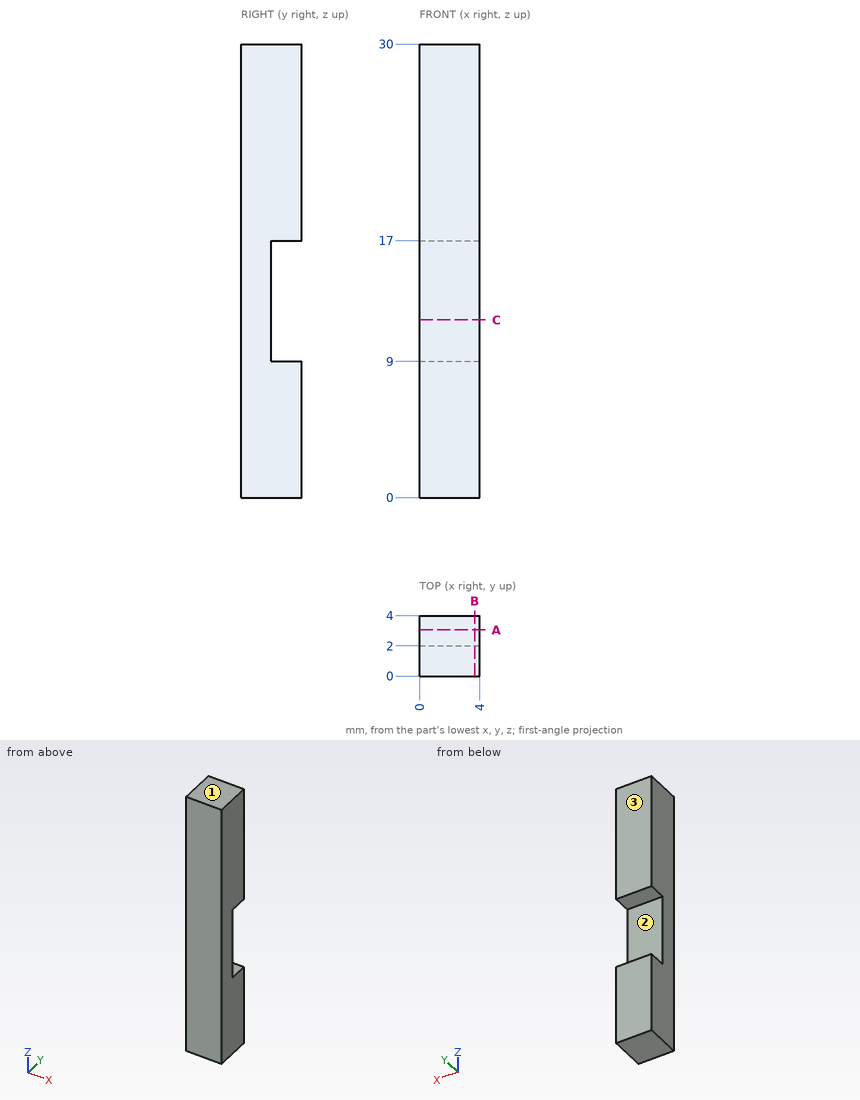
The figure shows three views and two pictorial views of one solid part (mm, origin at its lowest corner). Answer the questions. Coordinates: 2 decimals unless noted, no trailing zeros. Write each loop counter-clockwise with the first axis right and the second up, starting at its lowest first coordinate (ties: lowest second). Pieces come first, ordered by that corner, then holes. Notation, with made-up numbers: (-38, -31) -> (-26, -31) arc R15 cw to (-26, -12) -> close; hole circle Ø6 at (19, 46.5). An arc over 180 degrees is marked (long way). Return JSON: item names as keys, results as strings.
(1) The part is cut by section A-A on y = 3.05. Give the vertices of the cut face in (x, z), then the cut area to 3 significant figures.
Answers below:
{"outline": "(0, 0) -> (4, 0) -> (4, 9) -> (0, 9) -> close; (0, 17) -> (4, 17) -> (4, 30) -> (0, 30) -> close", "area": "88.0 mm^2"}
(2) The part is cut by section B-B on x = 3.65. Give the vertices of the cut face in (y, z).
Answers below:
{"outline": "(0, 0) -> (4, 0) -> (4, 9) -> (2, 9) -> (2, 17) -> (4, 17) -> (4, 30) -> (0, 30) -> close"}
(3) For a pull along Z with two mould halves and no side action, classify the marked faces 1, 2 and 3 as pulls with the +Z half, pulls with the -Z half, needs draft (parallel to the pull), parting line crosses it, or undercut.
Answers below:
{"face 1": "pulls with the +Z half", "face 2": "undercut", "face 3": "needs draft"}
(4) The part is cut by section C-C on z = 11.75. Give the vertices of the cut face in (x, y), then the cut area to 3 significant figures.
Answers below:
{"outline": "(0, 0) -> (4, 0) -> (4, 2) -> (0, 2) -> close", "area": "8.00 mm^2"}
(5) This flat-tipped pin is pushed along its axis until it touches: P1, Ø2, axis at x = 1.5, z = 13, coming from the +Y side. Where does it stop, or does it pass through?
Answers below:
{"P1": "y = 2"}
(6) Consider line 1 along Z through (x, y) = (0.75, 2.45); line 2 along Y through (x, z) = (1.3, 12). Determine where each line is inside the solid, lowest interval first. Write a range as from..to.
Answers below:
{"line 1": "0..9, 17..30", "line 2": "0..2"}
